Verification items for the finished model (mm, model axes). Give positions to 0.01 mm unless a question says otherwise; leave off trailing zeros. Order: outer loops, then holes, each group sorted by start corner. A loop starts at its lowest first (then second) coordinate and runs counter-clockwise, first axis right, second up.
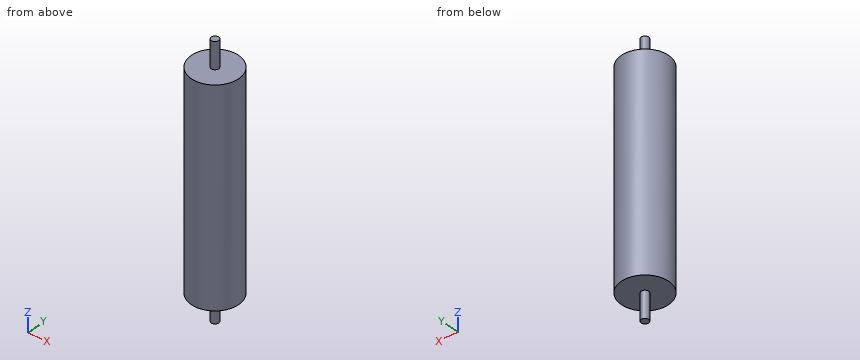
Autodesk Inventor part; units mm, degrees
ref_plane "YZ Plane" through (0, 0, 0) normal (1, 0, 0) x (0, 1, 0)
ref_plane "XZ Plane" through (0, 0, 0) normal (0, 1, 0) x (-1, 0, 0)
ref_plane "XY Plane" through (0, 0, 0) normal (0, 0, 1) x (1, 0, 0)
sketch "Sketch1" plane through (0, 0, 0) normal (0, 1, 0) x (-1, 0, 0)
  line L0 (0, 25) -> (0, -25)
  line L1 (0, 25) -> (0.7, 25)
  line L2 (0.7, 25) -> (0.7, 20)
  line L3 (0.7, 20) -> (4.5, 20)
  line L4 (4.5, 20) -> (4.5, -20)
  line L5 (4.5, -20) -> (0.7, -20)
  line L6 (0.7, -20) -> (0.7, -25)
  line L7 (0.7, -25) -> (0, -25)
  point P0 (0, 0)
  point P1 (0, 0)
  dimension "d0" = 9
  dimension "d1" = 1.4
  dimension "d2" = 5
  dimension "d3" = 40
revolve "Revolution1" add sketch "Sketch1" angle 360 about axis through (0, 0, 25) along (0, 0, -1)
properties part number "15kOhmResistor"
(1) Go/stop test with flat-tipped pins: pin 1 (3 mm diameter, centred on y = -3, z = 1, fed in from +X); pin 2 (1 mm diameter, centred on x = 2.5, z = 16, fed in from -Y); pin 3 (1.5 mm diameter, centred on x = -2, y = -1, fed in from -Z). Record where each tip stops, or that it passes through.
Solved:
pin 1: stops at x = 4.24
pin 2: stops at y = -4.03
pin 3: stops at z = -20
(2) Scan lines: line 1 (Z direction, x = 3, y = -1.5); line 2 (X direction, y = -2.25, z = 16); line 3 (X direction, y = 1, z = -0.5). Record each from-to range of solid material in increasing order.
Solved:
line 1: z = -20 to 20
line 2: x = -3.9 to 3.9
line 3: x = -4.39 to 4.39
(3) Section check D-D, the plane x = 2.75. Enter the section's corners in (y, z).
Solved:
outline: (-3.56, -20) - (3.56, -20) - (3.56, 20) - (-3.56, 20) - close
(4) Section check C-C, the plane z = -12.5. Enter the section's corners in (x, y).
Solved:
outline: circle Ø9 at (0, 0)
(5) Section check A-A, the plane x = 0. Enter the section's corners in (y, z).
Solved:
outline: (-4.5, -20) - (-0.7, -20) - (-0.7, -25) - (0.7, -25) - (0.7, -20) - (4.5, -20) - (4.5, 20) - (0.7, 20) - (0.7, 25) - (-0.7, 25) - (-0.7, 20) - (-4.5, 20) - close
